Build history of the part. All positions in model axes, mm. Give positions to 0.01 mm unless a question says otherwise; leave off trailing zeros. Write each loop counter-clockwise with the first axis right and the second up, starting at its lowest first coordinate (ties: lowest second). Pieces come first, ordered by that corner, then holes. Notation, with made-up numbers: (-36.75, 56.25) -> (11.25, 56.25) arc R6 ccw to (11.25, 64.25) -> close; hole circle Ø1 at (21.25, -31.5). An arc over 180 degrees is marked (long way). Write item = value, one per line. Start each with the question number.
Q1. Saw through at D-D, the plane y = 6.25. List the corners of the cut face in (x, z) (3 decimals), then the cut area to 3 significant figures.
Q2. Wall check: line 1 (Y direction, x = -12.7, z = 1.5); line 2 (X direction, y = -9.5, z = 3.5); line 3 (Y direction, x = -14, z = -3.25). Give the ranges that are in metal, low to high.
Q3. Mould opens along Z. For faces 1 (the face through (-1, 0, 9.525)), 2 (the face through (26.35, 0.18, 3.74)), 3 (the face through (-1, -12.7, 2)) say: pulls with the +Z half, pulls with the -Z half, needs draft (parallel to the pull), parting line crosses it, or undercut.
Q4. Saw through at C-C, the plane z = -4.75. List the corners of the cut face in (x, y).
Q5. Saw through at A-A, the plane x = -12.7. List the corners of the cut face in (y, z) (3 decimals), then the cut area to 3 significant figures.
Q6. Saw through at B-B, the plane y = 1. List the corners of the cut face in (x, z) (1 decimal), then the cut area to 3 significant figures.
from build123d import *

# Parameters (mm, degrees)
SKETCH1_W              = 76.2
SKETCH1_H              = 19.05
BOSS_EXTRUDE1_DEPTH    = 12.7
F_8_32_TAPPED_HOLE1_D  = 3.4544
F_10_CLEARANCE_HOLE1_D = 4.9784


with BuildPart() as part:
    # Sketch1 → Boss-Extrude1 (new, symmetric)
    with BuildSketch(Plane(origin=(0, 0, 0), x_dir=(1, 0, 0), z_dir=(0, 1, 0))):
        Rectangle(SKETCH1_W, SKETCH1_H)
    extrude(amount=BOSS_EXTRUDE1_DEPTH, both=True)

    # #8-32 Tapped Hole1 (through all)
    with Locations(Plane(origin=(-24.638, -12.7, 3.9624), x_dir=(0, 0, -1), z_dir=(0, -1, 0))):
        with Locations((0, 0), (5.5626, 24.638), (0, 49.276)):
            Hole(F_8_32_TAPPED_HOLE1_D / 2)

    # #10 Clearance Hole1 (through all)
    with Locations(Plane(origin=(0, 0, -9.525), x_dir=(-1, 0, 0), z_dir=(0, 0, -1))):
        with Locations((-12.7, 0), (12.7, 0)):
            Hole(F_10_CLEARANCE_HOLE1_D / 2)


solid = part.part
Report:
q1.outline = (-38.1, -9.525) -> (38.1, -9.525) -> (38.1, 9.525) -> (-38.1, 9.525) -> close; hole circle Ø3.454 at (-24.638, 3.962); hole circle Ø3.454 at (0, -1.6); hole circle Ø3.454 at (24.638, 3.962)
q1.area = 1,420 mm2
q2.line_1 = -12.7 to -2.49, 2.49 to 12.7
q2.line_2 = -38.1 to -26.3, -22.97 to 22.97, 26.3 to 38.1
q2.line_3 = -12.7 to -2.12, 2.12 to 12.7
q3.face_1 = pulls with the +Z half
q3.face_2 = undercut
q3.face_3 = needs draft
q4.outline = (-38.1, -12.7) -> (38.1, -12.7) -> (38.1, 12.7) -> (-38.1, 12.7) -> close; hole circle Ø4.98 at (-12.7, 0); hole circle Ø4.98 at (12.7, 0)
q5.outline = (-12.7, -9.525) -> (-2.489, -9.525) -> (-2.489, 9.525) -> (-12.7, 9.525) -> close; (2.489, -9.525) -> (12.7, -9.525) -> (12.7, 9.525) -> (2.489, 9.525) -> close
q5.area = 389 mm2
q6.outline = (-38.1, -9.5) -> (-15, -9.5) -> (-15, 9.5) -> (-38.1, 9.5) -> close; (-10.4, -9.5) -> (10.4, -9.5) -> (10.4, 9.5) -> (-10.4, 9.5) -> close; (15, -9.5) -> (38.1, -9.5) -> (38.1, 9.5) -> (15, 9.5) -> close; hole circle Ø3.5 at (-24.6, 4); hole circle Ø3.5 at (0, -1.6); hole circle Ø3.5 at (24.6, 4)
q6.area = 1,250 mm2
